Can you work these out from the model? Positions are in its coordinate system, mm. A direction names the side the tool comes from. Coordinates: 2 decimals unless noted, no trailing zeros. Loops run counter-clockwise (first coordinate to the right, second up) from the corner with the lowest first, then second, coordinate; pieces in that order, holes last.
```python
from build123d import *

# Parameters (mm, degrees)
F0_W     = 470
F0_H     = 1084
F1_DEPTH = 225
F2_R     = 60
F3_DEPTH = 70


with BuildPart() as f1:
    # F0 (on Front) → F1 (new body, symmetric)
    with BuildSketch(Plane.XZ):
        Rectangle(F0_W, F0_H)
    extrude(amount=F1_DEPTH, both=True)

    # F2 (on face) → F3 (join)
    with BuildSketch(Plane.XZ.offset(225)):
        with Locations((-115.5, 392)):
            Circle(F2_R)
        with Locations((-115.5, -327)):
            Circle(F2_R)
        with Locations((115.5, 392)):
            Circle(F2_R)
        with Locations((115.5, -327)):
            Circle(F2_R)
    extrude(amount=F3_DEPTH)


solid = f1.part
```
(1) If I drill on probe 1 along Y at (x, z) = (-159.5, 494); probe 2 along Z at (x, y) = (-64, -238.5), over which ranges is the centre line in solid material (lowest first)?
Check values:
probe 1: y = -225 to 225
probe 2: z = -357.79 to -296.21, 361.21 to 422.79
(2) Which directions (+Z, -Z, +X, -X, +Y, -Y) give clear straight access to the entire face, cutting with the end or side of a thin tool? Please do faces 4 (the flat face through (-116, -295, 393)), 5 (the cylindrical face through (102.493, -259.51, -385.573)).
Check values:
face 4: +Z, -Z, +X, -X, -Y
face 5: -Y
(3) I want a section at A-A on x = -115.5. Write out the boundary of the cut face in (y, z), then the cut area to 3 significant figures.
Check values:
outline: (-295, -387) - (-225, -387) - (-225, -542) - (225, -542) - (225, 542) - (-225, 542) - (-225, 452) - (-295, 452) - (-295, 332) - (-225, 332) - (-225, -267) - (-295, -267) - close
area: 505,000 mm2
(4) I want a section at B-B on z = -327. Write out the boundary of the cut face in (x, y).
Check values:
outline: (-235, -225) - (-175.5, -225) - (-175.5, -295) - (-55.5, -295) - (-55.5, -225) - (55.5, -225) - (55.5, -295) - (175.5, -295) - (175.5, -225) - (235, -225) - (235, 225) - (-235, 225) - close
(5) I want a section at C-C on z = 7. Write out the boundary of the cut face in (x, y).
Check values:
outline: (-235, -225) - (235, -225) - (235, 225) - (-235, 225) - close
(6) If we mould it in two halves opening along X, with no side actions, what happens to faces 1 (the flat face through (235, -3, -8)), 2 (the flat face through (-116, -295, -326)), 3 (the cylindrical face through (102.493, -259.51, 333.427))? For each: released by +X, released by -X, zero draft, split by the parting line, or undercut.
Check values:
face 1: released by +X
face 2: zero draft
face 3: undercut
(7) I want a section at D-D on x = -14.5. Write out the boundary of the cut face in (y, z), then the cut area to 3 significant figures.
Check values:
outline: (-225, -542) - (225, -542) - (225, 542) - (-225, 542) - close
area: 488,000 mm2
(8) I'm going to push a flat-ended pin straight in: pin 1 (12 mm diameter, centred on x = 80.5, z = 203.5, fed in from -Y). Where does the tip first touch, or does it pass through?
Check values:
pin 1: stops at y = -225
